Build history of the part. All positions in model axes, mm. Round coordinates to 2 decimals unless told otherwise and drop trailing zeros. Write each loop counter-clockwise with the first axis right and the second up, starting at its lowest first coordinate (ties: lowest second). Pieces come first, ordered by that corner, then holes.
Autodesk Inventor part; units mm, degrees
ref_plane "YZ Plane" through (0, 0, 0) normal (1, 0, 0) x (0, 1, 0)
ref_plane "XZ Plane" through (0, 0, 0) normal (0, 1, 0) x (-1, 0, 0)
ref_plane "XY Plane" through (0, 0, 0) normal (0, 0, 1) x (1, 0, 0)
sketch "Sketch1" plane through (0, 0, 0) normal (0, 1, 0) x (-1, 0, 0)
  circle A0 centre (0, 0) radius 73.025
  dimension "d4" = 146.05
extrude "Extrusion1" add sketch "Sketch1" against normal blind 6.35
sketch "Sketch5" plane through (0, 0, 0) normal (0, 1, 0) x (1, 0, 0)
  circle A0 centre (0, 0) radius 63.5 construction
  circle A1 centre (-63.5, 0) radius 3.3782
  circle A2 centre (-51.3726, -37.3244) radius 3.3782
  circle A3 centre (-19.6226, -60.3921) radius 3.3782
  circle A4 centre (19.6226, -60.3921) radius 3.3782
  circle A5 centre (51.3726, -37.3244) radius 3.3782
  circle A6 centre (63.5, 0) radius 3.3782
  circle A7 centre (51.3726, 37.3244) radius 3.3782
  circle A8 centre (19.6226, 60.3921) radius 3.3782
  circle A9 centre (-19.6226, 60.3921) radius 3.3782
  circle A10 centre (-51.3726, 37.3244) radius 3.3782
  dimension "d17" = 127
  dimension "d18" = 6.7564
  dimension "d21" = 360
extrude "Extrusion4" cut sketch "Sketch5" against normal through all
properties part number "SupportPlateForWater" material "PET Plastic"
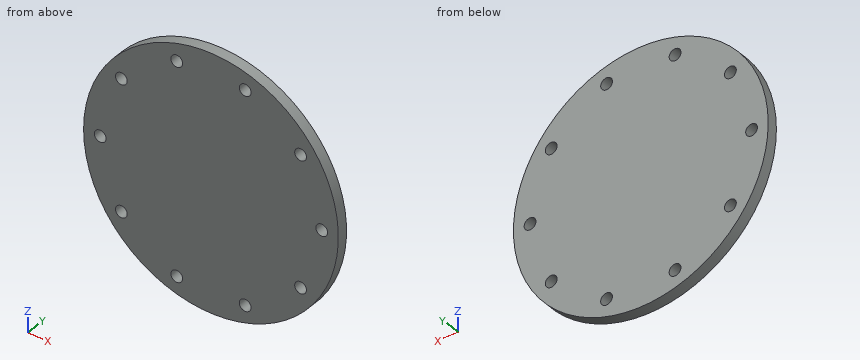
1) Pin check, flat tips, straight feed: pin 1 Ø1 at (y, z) = (-3.5, -56) entering from -X; pin 2 Ø1.5 at (y, z) = (-2, 43.5) entering from +X. Stop position of each tip, or through.
Results:
pin 1: stops at x = -47.46
pin 2: stops at x = 59.2
2) Slice it at C-C (x = -63.5). Write the cut outline in (y, z), plus the area to 3 significant figures.
Results:
outline: (-6.35, -36.06) - (0, -36.06) - (0, -3.38) - (-6.35, -3.38) - close; (-6.35, 3.38) - (0, 3.38) - (0, 36.06) - (-6.35, 36.06) - close
area: 415 mm2
3) Slice it at A-A (z = 0). Write the cut outline in (x, y) (3 decimals).
Results:
outline: (-73.025, -6.35) - (-66.878, -6.35) - (-66.878, 0) - (-73.025, 0) - close; (-60.122, -6.35) - (60.122, -6.35) - (60.122, 0) - (-60.122, 0) - close; (66.878, -6.35) - (73.025, -6.35) - (73.025, 0) - (66.878, 0) - close
4) Slice it at B-B (y = -3.5). Count the separate pieces of the cut face and the enclosed holes in it, plus the area to 3 significant figures.
Results:
separate pieces: 1
enclosed holes: 10
area: 16,400 mm2
5) Slice it at D-D (x = -31.5). Write the cut outline in (y, z), plus the area to 3 significant figures.
Results:
outline: (-6.35, -65.88) - (0, -65.88) - (0, 65.88) - (-6.35, 65.88) - close
area: 837 mm2
6) Wall check: L1, parallel to X at y = -4.25, z = 40; L2, parallel to Z at x = 51, y = -1.5; L3, parallel to X at y = -2, z = -2. Give the ranges that are in metal, low to high.
Results:
L1: x = -61.1 to -53.43, -49.31 to 49.31, 53.43 to 61.1
L2: z = -52.27 to -40.68, -33.97 to 33.97, 40.68 to 52.27
L3: x = -73 to -66.22, -60.78 to 60.78, 66.22 to 73
